Can you work these out from the drawing? Everything is in mm from the part's minimum corner. A direction names the side the tool comes from. Coordinates: 2 decimals unless noted, no trailing zeros. Order: outer loops, then holes, each group sorted by start corner. A loop starts at its lowest first (then second) coordinate and runs counter-clockwise, first axis right, second up. Notation, with made-up numbers: M 8,11.5 L 36,11.5 A22 cw 36,32.5 Z; hole C -4.5,-0.5 d11. An arc over 180 degrees is marked long. Answer as a JSON object with one key per item and string values.
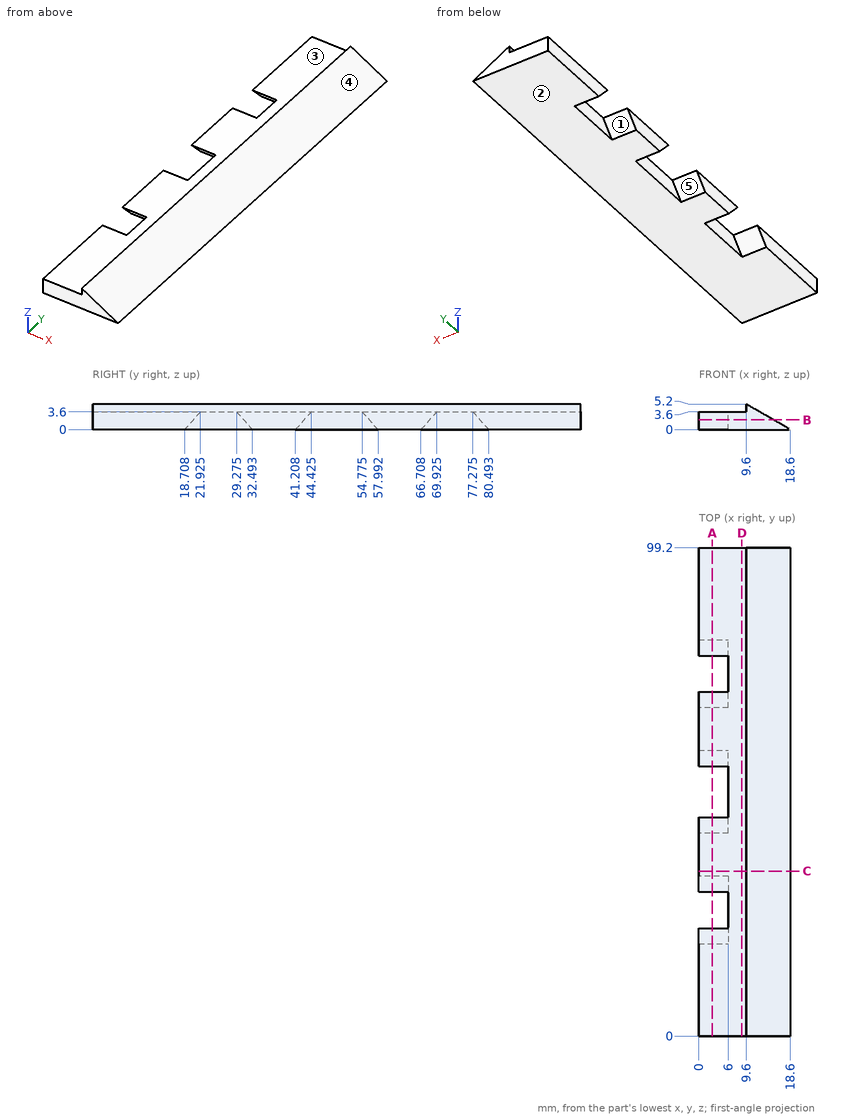
Item 1: Please list where these lines run through material, in increasing order: line 1 (Y direction, x = 2.75, z = 0.55); line 2 (Z direction, x = 6, y = 92); line 3 (X direction, y = 68, z = 1.1) (1 decimal).
Answers follow:
{"line 1": "y = 0 to 19.2, 32 to 41.7, 57.5 to 67.2, 80 to 99.2", "line 2": "z = 0 to 3.6", "line 3": "x = 6 to 16.7"}
Item 2: I want a section at A-A, the plane x = 2.75. Write out the boundary of the cut face in (y, z) (1 decimal).
Answers follow:
{"outline": "M 0,0 L 18.7,0 L 21.9,3.6 L 0,3.6 Z; M 29.3,3.6 L 32.5,0 L 41.2,0 L 44.4,3.6 Z; M 54.8,3.6 L 58,0 L 66.7,0 L 69.9,3.6 Z; M 77.3,3.6 L 80.5,0 L 99.2,0 L 99.2,3.6 Z"}
Item 3: I want a section at B-B, the plane z = 2. Write out the boundary of the cut face in (x, y) (1 decimal).
Answers follow:
{"outline": "M 0,0 L 15.1,0 L 15.1,99.2 L 0,99.2 L 0,78.7 L 6,78.7 L 6,68.5 L 0,68.5 L 0,56.2 L 6,56.2 L 6,43 L 0,43 L 0,30.7 L 6,30.7 L 6,20.5 L 0,20.5 Z"}
Item 4: Which directions (+Z, -Z, +X, -X, +Y, -Y) give clear straight access to the entire face, cutting with the end or side of a thin tool? Please do the marked faces 1, 2 and 3.
Answers follow:
{"face 1": "-Z, -X", "face 2": "-Z, +X, -X, +Y, -Y", "face 3": "+Z, -X, +Y, -Y"}
Item 5: I'm going to push flat-ended pins straight in: pin 1 (5 mm diameter, centred on x = 3.5, y = 62.5, fed in from +Z); pin 2 (4 mm diameter, centred on x = 13.5, y = 79, fed in from +Z); pin 3 (1.1 mm diameter, centred on y = 48.5, z = 2.5, fed in from -X). Where does each tip first touch, or does it pass through?
Answers follow:
{"pin 1": "stops at z = 3.6", "pin 2": "stops at z = 4.1", "pin 3": "stops at x = 6"}
Item 6: I want a section at D-D, the plane x = 8.75. Write out the boundary of the cut face in (y, z), plus the area to 3 significant figures.
Answers follow:
{"outline": "M 0,0 L 99.2,0 L 99.2,3.6 L 0,3.6 Z", "area": "357 mm^2"}
Item 7: I want a section at C-C, the plane y = 33.5. Write out the boundary of the cut face in (x, z).
Answers follow:
{"outline": "M 0,0 L 18.6,0 L 9.6,5.2 L 9.6,3.6 L 0,3.6 Z"}
Item 8: If we mould it in two halves opening along Y, with no side actions, what happens to the marked faces 4 and 5? For each: pulls with the +Y half, pulls with the -Y half, needs draft (parallel to the pull), parting line crosses it, or undercut.
Answers follow:
{"face 4": "needs draft", "face 5": "undercut"}
